Verification items for the finished model (mm, model axes). Face numbers are marked on the shaded views. A direction names the side the tool comes from. Coordinates: 2 decimals unless noted, no trailing zeros. Order: outer loops, then holes, each group sorted by start corner. A loop starts at its lowest first (then second) coordinate and runs counter-clockwise, first axis right, second up.
Q1. Draft check along X on the marked faces 3, 4 and 5. Enter one of: pulls with the +X half, pulls with the -X half, needs draft (parallel to the pull), parting line crosses it, or undercut.
Q2. Cross-section at C-C, the plane z = -21.75. Record the boundary of the cut face in (x, y) (3 decimals), and give its area (3 significant figures).
Q3. Thickness scan on line 1 (X direction, y = -21, z = -20.5); line 2 (Z direction, x = 21.5, y = -7); line 3 (Y direction, x = 12.5, z = -20.75). Record the ranges inside material, lowest first.
Q4. Cross-section at A-A, the plane x = 0. Record the boundary of the cut face in (y, z), and give its area (3 significant figures).
Q5. Set-up check for the marked faces 1 and 2: record each of +Z, -Z, +X, -X, +Y, -Y from which the full face is reachable in a straight line by a thin tool's end or side.
Q6. Cross-section at D-D, the plane x = -23.75. Record the boundary of the cut face in (y, z), and give its area (3 significant figures).
Q7. Cross-section at B-B, the plane y = 0. Record the boundary of the cut face in (x, z).
Q8. Depth check by flat-ended pin: P1, Ø4.5, axis at x = 0, z = -10.2, coming from the +Y side; P2, Ø3, axis at x = -10.5, z = -16.5, coming from the -Y side; P3, Ø8.5, axis at x = -23.75, y = 0, coming from the +Z side; P4, Ø3, axis at x = 11.88, y = -20.57, coming from the -Z side. Enter the tip coordinate at first touch or a pass-through.
from build123d import *

# Parameters (mm, degrees)
SKETCH2_R               = 2.6
CUT_EXTRUDE1_DEPTH      = 48.098619937
CUT_EXTRUDE2_REACH      = 49.099
CUT_EXTRUDE2_END_RADIUS = 12
SKETCH3_R               = 2.75


with BuildPart() as part:
    # Sketch1 → Revolve1 (revolve)
    with BuildSketch(Plane(origin=(0, 0, 0), x_dir=(1, 0, 0), z_dir=(0, 1, 0)), mode=Mode.PRIVATE) as revolve1_sk:
        Polygon((-5, 24.6), (-28.4, 24.6), (-28.4, 18.6), (-12, 18.6), (-12, 0), (-5, 0), align=None)
    revolve(revolve1_sk.sketch.rotate(Axis((0, 0, 0), (0, 0, -1)), 180), axis=Axis((0, 0, 0), (0, 0, -1)))

    # Sketch2 → Cut-Extrude1 (cut, through all)
    with BuildSketch(Plane(origin=(0, 0, -24.6), x_dir=(-1, 0, 0), z_dir=(0, 0, -1))):
        with Locations((-23.75, 0)):
            Circle(SKETCH2_R)
        with Locations((-11.875, 20.56810334)):
            Circle(SKETCH2_R)
        with Locations((11.875, 20.56810334)):
            Circle(SKETCH2_R)
        with Locations((23.75, 0)):
            Circle(SKETCH2_R)
        with Locations((11.875, -20.56810334)):
            Circle(SKETCH2_R)
        with Locations((-11.875, -20.56810334)):
            Circle(SKETCH2_R)
    extrude(amount=-CUT_EXTRUDE1_DEPTH, mode=Mode.SUBTRACT)

    # Cut-Extrude2: up to this cylinder (the profile starts inside it)
    cut_extrude2_end = Plane(origin=(0, 0, -10.2), z_dir=(0, 0, 1)) * Cylinder(CUT_EXTRUDE2_END_RADIUS, 123.198, mode=Mode.PRIVATE)
    # Sketch3 → Cut-Extrude2 (cut, up to the surface)
    with BuildSketch(Plane(origin=(0, 0, 0), x_dir=(1, 0, 0), z_dir=(0, 1, 0)), mode=Mode.PRIVATE) as cut_extrude2_sk1:
        with Locations(Location((0, 10.2, 0), (0, 0, 270))):
            Circle(SKETCH3_R)
    cut_extrude2_tool1 = extrude(cut_extrude2_sk1.sketch, amount=-CUT_EXTRUDE2_REACH, mode=Mode.PRIVATE) & cut_extrude2_end
    add(cut_extrude2_tool1.solids().sort_by_distance((0, 0, -10.2))[0], mode=Mode.SUBTRACT)


solid = part.part
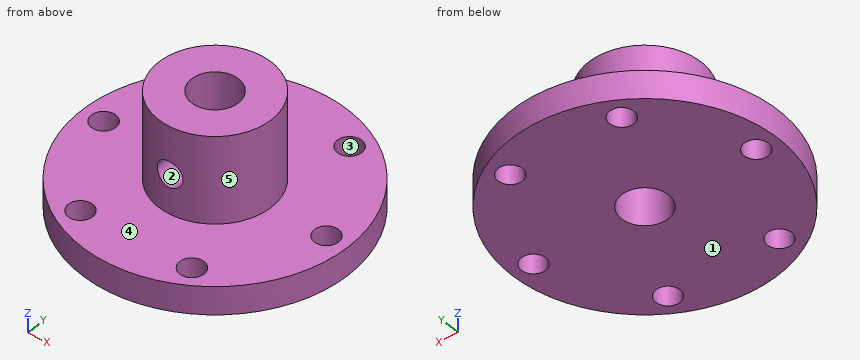
Check values:
1. face 3: undercut
1. face 4: needs draft
1. face 5: parting line crosses it
2. outline: circle Ø56.8 at (0, 0); hole circle Ø5.2 at (-23.75, 0); hole circle Ø5.2 at (-11.875, -20.568); hole circle Ø5.2 at (-11.875, 20.568); hole circle Ø10 at (0, 0); hole circle Ø5.2 at (11.875, -20.568); hole circle Ø5.2 at (11.875, 20.568); hole circle Ø5.2 at (23.75, 0)
2. area: 2,330 mm2
3. line 1: x = -19.12 to -14.44, -9.31 to 9.31, 14.44 to 19.12
3. line 2: z = -24.6 to -18.6
3. line 3: y = -25.5 to -23.09, -18.04 to 18.04, 23.09 to 25.5
4. outline: (-28.4, -24.6) - (-5, -24.6) - (-5, -12.95) - (-12, -12.95) - (-12, -18.6) - (-28.4, -18.6) - close; (-12, -7.45) - (-5, -7.45) - (-5, 0) - (-12, 0) - close; (5, -24.6) - (28.4, -24.6) - (28.4, -18.6) - (12, -18.6) - (12, 0) - (5, 0) - close
4. area: 503 mm2
5. face 1: -Z, +X, -X, +Y, -Y
5. face 2: -Y
6. outline: (-15.57, -24.6) - (-2.6, -24.6) - (-2.6, -18.6) - (-15.57, -18.6) - close; (2.6, -24.6) - (15.57, -24.6) - (15.57, -18.6) - (2.6, -18.6) - close
6. area: 156 mm2
7. outline: (-28.4, -24.6) - (-26.35, -24.6) - (-26.35, -18.6) - (-28.4, -18.6) - close; (-21.15, -24.6) - (-5, -24.6) - (-5, 0) - (-12, 0) - (-12, -18.6) - (-21.15, -18.6) - close; (5, -24.6) - (21.15, -24.6) - (21.15, -18.6) - (12, -18.6) - (12, 0) - (5, 0) - close; (26.35, -24.6) - (28.4, -24.6) - (28.4, -18.6) - (26.35, -18.6) - close
8. P1: stops at y = 12
8. P2: stops at y = -7.94
8. P3: stops at z = -18.6
8. P4: passes through
